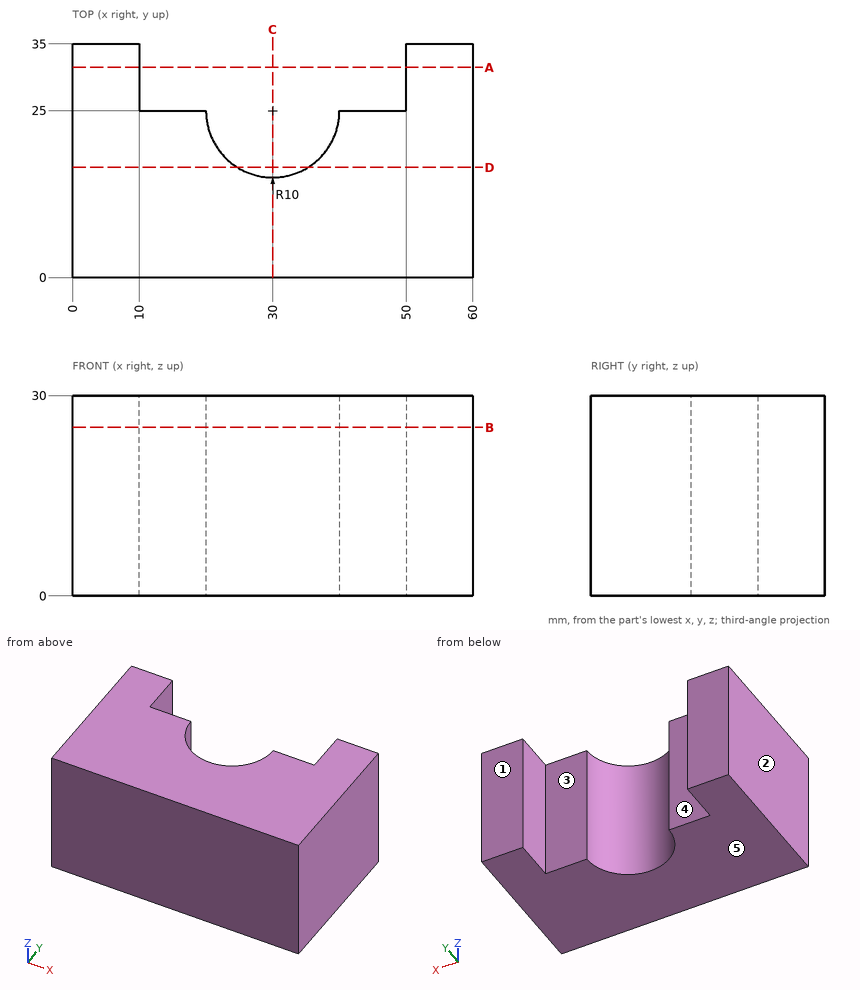
Geometry: see drawing. Coordinates: mm, zero at the bounding-box minimum. A direction names the side the tool comes from. Give positions to 0.01 mm unless a question says otherwise; leave off trailing zeros. Loops run counter-clockwise (first coordinate to the right, second up) from the corner with the lowest first, then second, coordinate; pieces in that order, holes last. Notation, with made-up numbers: (54.25, 82) -> (78.25, 82) arc R17 ccw to (78.25, 107) -> close; hole circle Ø9 at (28, 87.25). An arc over 180 degrees is marked (long way). Put each result on its own line as item: value.
1. Pull-direction query (X, two-part tool) for the marked faces 1, 2 and 3; classes: released by +X, released by -X, zero draft, split by the parting line, or undercut.
Taken from the geometry:
face 1: zero draft
face 2: released by -X
face 3: undercut
2. Cut plane C-C (x = 30). Return the cut outline in (y, z), plus the area to 3 significant figures.
Taken from the geometry:
outline: (0, 0) -> (15, 0) -> (15, 30) -> (0, 30) -> close
area: 450 mm2
3. Pin query (flat end, axial travel): P1, Ø10, axis at x = 17.5, z = 18.5, coming from the -Y side; P2, Ø6, axis at x = 39.5, z = 26.5, coming from the +Y side. Return the tip coordinate at first contact, or that it passes through.
Taken from the geometry:
P1: stops at y = 0
P2: stops at y = 25
4. Cut plane B-B (z = 25.25). Return the cut outline in (x, y), plus the area to 3 significant figures.
Taken from the geometry:
outline: (0, 0) -> (60, 0) -> (60, 35) -> (50, 35) -> (50, 25) -> (40, 25) arc R10 cw to (20, 25) -> (10, 25) -> (10, 35) -> (0, 35) -> close
area: 1,540 mm2
5. Set-up query: the marked faces 4 and 5. Return all of +Z, -Z, +X, -X, +Y, -Y with unobstructed straight access to the full face (end or side cutting, diameter ignored); none if empty.
Taken from the geometry:
face 4: +Z, -Z, +Y
face 5: -Z, +X, -X, +Y, -Y
6. Cut plane D-D (y = 16.5). Return the cut outline in (x, z), plus the area to 3 significant figures.
Taken from the geometry:
outline: (0, 0) -> (24.73, 0) -> (24.73, 30) -> (0, 30) -> close; (35.27, 0) -> (60, 0) -> (60, 30) -> (35.27, 30) -> close
area: 1,480 mm2
7. Cut plane A-A (y = 31.5). Return the cut outline in (x, z).
Taken from the geometry:
outline: (0, 0) -> (10, 0) -> (10, 30) -> (0, 30) -> close; (50, 0) -> (60, 0) -> (60, 30) -> (50, 30) -> close
8. Ray query, line 1 along X through (y, z) = (28.5, 4.5); line 2 along Y through (x, z) = (10.5, 10); line 3 along X through (y, z) = (24, 21). Return the intervals inside material, ascending. Write a range as [from, to].
Taken from the geometry:
line 1: x = [0, 10], [50, 60]
line 2: y = [0, 25]
line 3: x = [0, 20.05], [39.95, 60]
